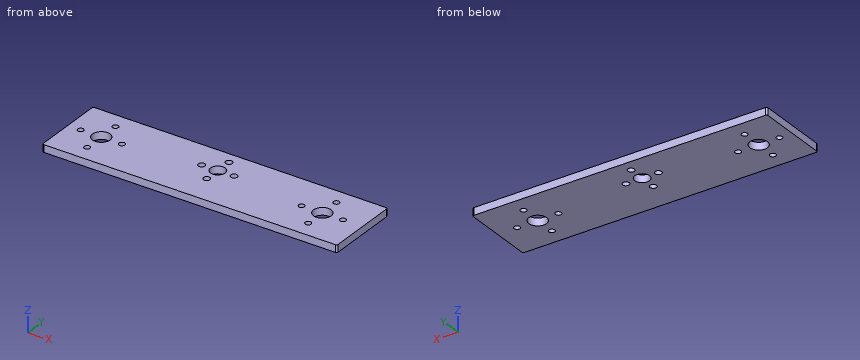
Autodesk Inventor part; units mm, degrees
ref_plane "YZ Plane" through (0, 0, 0) normal (1, 0, 0) x (0, 1, 0)
ref_plane "XZ Plane" through (0, 0, 0) normal (0, 1, 0) x (-1, 0, 0)
ref_plane "XY Plane" through (0, 0, 0) normal (0, 0, 1) x (1, 0, 0)
sketch "Sketch1" plane through (0, 0, 0) normal (0, 0, 1) x (1, 0, 0)
  line L0 (199.9787, 50.2308) -> (-0.0213, 50.2308)
  circle A0 centre (172.7248, 39.2308) radius 2
  circle A1 centre (158.7248, 25.2308) radius 2
  circle A2 centre (172.7248, 11.2308) radius 2
  circle A3 centre (186.7248, 25.2308) radius 2
  circle A4 centre (22.7248, 39.2308) radius 2
  circle A5 centre (8.7248, 25.2308) radius 2
  circle A6 centre (22.7248, 11.2308) radius 2
  circle A7 centre (36.7248, 25.2308) radius 2
  circle A8 centre (97.7248, 31.2308) radius 5
  circle A9 centre (172.7248, 25.2308) radius 6
  circle A10 centre (22.7248, 25.2308) radius 6
  circle A11 centre (97.7248, 20.2308) radius 2.25
  circle A12 centre (86.7248, 31.2308) radius 2.25
  circle A13 centre (108.7248, 31.2308) radius 2.25
  circle A14 centre (97.7248, 42.2308) radius 2.25
  line L1 (-0.0213, 50.2308) -> (-0.0213, 0)
  line L2 (-0.0213, 0) -> (199.9787, 0)
  line L3 (199.9787, 0) -> (199.9787, 50.2308)
  point P0 (0, 0)
extrude "Extrusion1" add sketch "Sketch1" along normal blind 5
fillet "Fillet1" radius 1 1 edges at (199.9787, 50.2308, 2.5)
fillet "Fillet2" radius 1 1 edges at (199.9787, 0, 2.5)
fillet "Fillet3" radius 1 1 edges at (-0.0213, 0, 2.5)
fillet "Fillet4" radius 1 1 edges at (-0.0213, 50.2308, 2.5)
properties part number "print bed test strut"
Model file for the job. Use its own axes, mm. Coordinates: 2 decimals unless noted, no trailing zeros. One line per item, written item: value. Start each with the question number.
1. Probe line 1 (X direction, y = 21, z = 0.55); line 2 (X direction, y = 29.5, z = 1.1); line 3 (X direction, y = 28, z = 4.05). List the from-to ranges inside material, lowest first. Write a range as from..to.
2. Flat gauge pins, fed straight in: pin 1 (2.5 mm diameter, centred on x = 186.72, y = 25.23, fed in from -Z); pin 2 (5 mm diameter, centred on x = 27.5, y = 34.5, fed in from -Z). Where does each tip first touch, or does it go through?
3. Slice it at A-A (z = 1.8). Count the separate pieces of the cut face and the enclosed holes in it, plus the area to 3 significant figures.
Answers below:
1. line 1: x = -0.02..18.47, 26.98..95.61, 99.84..168.47, 176.98..199.98
1. line 2: x = -0.02..18.51, 26.94..85.29, 88.16..93.03, 102.42..107.29, 110.16..168.51, 176.94..199.98
1. line 3: x = -0.02..17.4, 28.05..93.91, 101.54..167.4, 178.05..199.98
2. pin 1: passes through
2. pin 2: stops at z = 0
3. separate pieces: 1
3. enclosed holes: 15
3. area: 9,580 mm^2
